from build123d import *

# Parameters (mm, degrees)
PAD_DEPTH    = 12
SKETCH001_R  = 19.5
PAD001_DEPTH = 61
SKETCH002_R  = 3.175
POCKET_DEPTH = 8


with BuildPart() as part:
    # Sketch → Pad (new body)
    with BuildSketch(Plane.XY):
        Polygon((-19, 19), (19, 19), (19, -19), (7, -19), (7, -31), (-7, -31), (-7, -19), (-19, -19), align=None)
    extrude(amount=PAD_DEPTH)

    # Sketch001 → Pad001 (join)
    with BuildSketch(Plane.XY):
        Circle(SKETCH001_R)
    extrude(amount=-PAD001_DEPTH)

    # Sketch002 (on Face6 of Pad001) → Pocket (cut)
    with BuildSketch(Plane.XZ.offset(31)):
        with Locations((0, 6)):
            Circle(SKETCH002_R)
    extrude(amount=-POCKET_DEPTH, mode=Mode.SUBTRACT)


solid = part.part
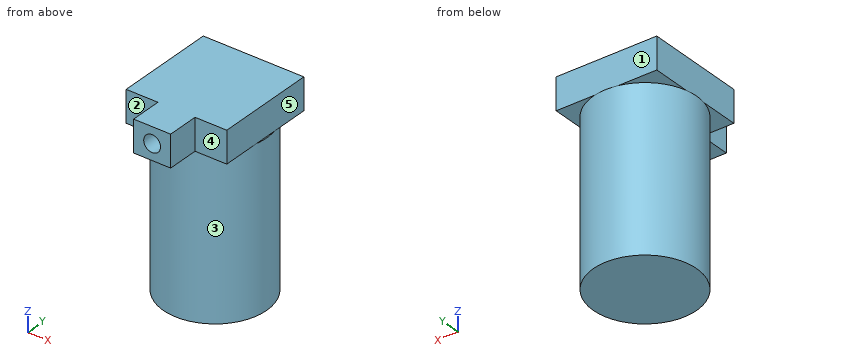
Geometry check sheet. Reference: the model listing, model coordinates, mm. Face numbers are marked on the shaded views. A direction names the side the tool comes from. Coordinates: 2 decimals unless noted, no trailing zeros. Order: outer loops, then holes, each group sorted by start corner. A loop starts at its lowest first (then second) coordinate and runs counter-clockwise, first axis right, second up. Notation, with made-up numbers: M -22.75,86 L 12.25,86 A27 cw 12.25,103 Z; hole C 15,-13 d10. An arc over 180 degrees is marked long. Use CSV: the item, a comma, the result in double quotes.
Item 1: Tool access check on the marked faces 1, 2, 3, 4 and 5. Record the directions out of +Z, -Z, +X, -X, +Y, -Y that give a thin tool (end or side, any length) a straight path to the whole face; none if there is none.
Returned:
face 1,"+Z, +X, -X, +Y"
face 2,"+Z, -Z, -X, -Y"
face 3,"-Z"
face 4,"+Z, -Z, +X, -Y"
face 5,"+Z, +X, +Y, -Y"
Item 2: Gauge pin test, flat ends, axial feed: pin 1 Ø12 at (x, z) = (-4, -21) entering from -Y; pin 2 Ø9.5 at (x, z) = (8.5, 6) entering from +Y; pin 3 Ø12 at (x, z) = (-15, 1) entering from -Y. Record the tip position at first contact, or that the pin passes through.
Returned:
pin 1,"stops at y = -19.5"
pin 2,"stops at y = 19"
pin 3,"stops at y = -19"
Item 3: Cross-section at B-B on z = 6. Record the cut outline in (x, y) (3 decimals), then the cut area to 3 significant figures.
Returned:
outline,"M -19,-19 L -7,-19 L -7,-31 L -3.175,-31 L -3.175,-23 L 3.175,-23 L 3.175,-31 L 7,-31 L 7,-19 L 19,-19 L 19,19 L -19,19 Z"
area,"1,560 mm2"
Item 4: Cross-section at A-A on x = 0. Record the cut outline in (y, z) (3 decimals), then the cut area to 3 significant figures.
Returned:
outline,"M -31,0 L -19.5,0 L -19.5,-61 L 19.5,-61 L 19.5,0 L 19,0 L 19,12 L -31,12 L -31,9.175 L -23,9.175 L -23,2.825 L -31,2.825 Z"
area,"2,930 mm2"
Item 5: Cross-section at D-D on z = -20. Record the cut outline in (x, y), then the cut area to 3 significant figures.
Returned:
outline,"C 0,0 d39"
area,"1,190 mm2"
Item 6: Cross-section at C-C on y = -8.5. Record the cut outline in (x, z), then the cut area to 3 significant figures.
Returned:
outline,"M -19,0 L -17.55,0 L -17.55,-61 L 17.55,-61 L 17.55,0 L 19,0 L 19,12 L -19,12 Z"
area,"2,600 mm2"
Item 7: Thickness scan on line 1 along Z through (x, y) = (0, -27) (3 decimals); line 2 along Y through (x, z) = (9.5, 4). Record the ranges inside material, lowest first.
Returned:
line 1,"z = 0 to 2.825, 9.175 to 12"
line 2,"y = -19 to 19"
